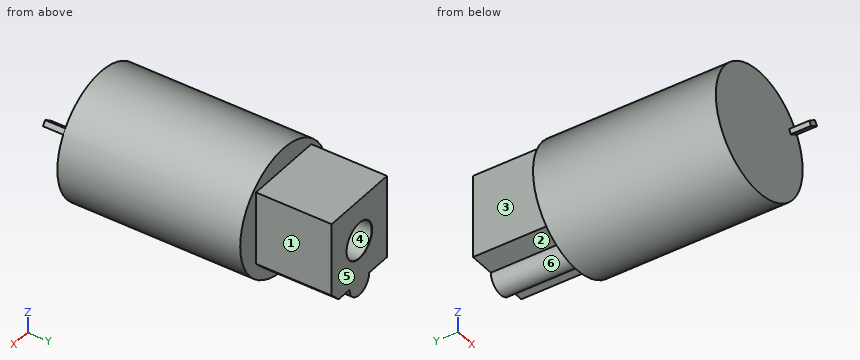
from build123d import *

# Parameters (mm, degrees)
ESBO_O1_R                              = 6.2
RESSALTO_EXTRUS_O1_DEPTH               = 18.1
RESSALTO_EXTRUS_O2_DEPTH               = 2
RESSALTO_EXTRUS_O3_DEPTH               = 7.5
CHANFRO1_SIZE                          = 1
FURO_DE_DI_METRO_3_6_3_6_1_D           = 3.6
FURO_DE_DI_METRO_3_6_3_6_1_DEPTH       = 10
FURO_DE_DI_METRO_3_6_3_6_1_CSINK_D     = 3.65
FURO_DE_DI_METRO_3_6_3_6_1_CSINK_ANGLE = 90
FURO_DE_DI_METRO_3_6_3_6_1_TIP         = 1.081549114


with BuildPart() as part:
    # Esboço1 → Ressalto-extrusão1 (new body)
    with BuildSketch(Plane(origin=(0, 0, 0), x_dir=(1, 0, 0), z_dir=(0, 1, 0))):
        Circle(ESBO_O1_R)
    extrude(amount=RESSALTO_EXTRUS_O1_DEPTH)

    # Esboço2 → Ressalto-extrusão2 (add)
    with BuildSketch(Plane(origin=(0, 0, 0), x_dir=(1, 0, 0), z_dir=(0, 1, 0))):
        with BuildLine():
            Line((4.5033321, -2.6), (5.369357503, -3.1))
            ThreePointArc((5.369357503, -3.1), (5.229026964, -3.331257572), (5.078742675, -3.556173905))
            Line((5.078742675, -3.556173905), (4.25959063, -2.982597469))
            ThreePointArc((4.25959063, -2.982597469), (4.385635518, -2.793957963), (4.5033321, -2.6))
        make_face()
    extrude(amount=-RESSALTO_EXTRUS_O2_DEPTH)

    # Esboço3 → Ressalto-extrusão3 (add)
    with BuildSketch(Plane(origin=(0, 18.1, 0), x_dir=(1, 0, 0), z_dir=(0, 1, 0))):
        with BuildLine():
            Line((1.4, 4.15), (3.95, 4.15))
            Line((3.95, 4.15), (3.95, -4.15))
            Line((3.95, -4.15), (-3.95, -4.15))
            Line((-3.95, -4.15), (-3.95, 4.15))
            Line((-3.95, 4.15), (-1.4, 4.15))
            ThreePointArc((-1.4, 4.15), (0, 5.55), (1.4, 4.15))
        make_face()
    extrude(amount=RESSALTO_EXTRUS_O3_DEPTH)

    # Chanfro1
    chanfro1_edges = [part.edges().sort_by_distance(p)[0] for p in [
        (3.95, 21.85, -4.15),
    ]]
    chamfer(chanfro1_edges, length=CHANFRO1_SIZE)

    # Furo de diâmetro Ø3.6 (3.6)1
    with Locations(Plane(origin=(0, 25.6, 0), x_dir=(1, 0, 0), z_dir=(0, 1, 0))):
        with Locations((0, 0)):
            CounterSinkHole(FURO_DE_DI_METRO_3_6_3_6_1_D / 2, FURO_DE_DI_METRO_3_6_3_6_1_CSINK_D / 2, depth=FURO_DE_DI_METRO_3_6_3_6_1_DEPTH, counter_sink_angle=FURO_DE_DI_METRO_3_6_3_6_1_CSINK_ANGLE)
            with Locations((0, 0, -(FURO_DE_DI_METRO_3_6_3_6_1_DEPTH + FURO_DE_DI_METRO_3_6_3_6_1_TIP / 2))):  # 118° drill point
                Cone(0, FURO_DE_DI_METRO_3_6_3_6_1_D / 2, FURO_DE_DI_METRO_3_6_3_6_1_TIP, mode=Mode.SUBTRACT)


solid = part.part
Part model, mm, in its own coordinate system. Face numbers are marked on the shaded views. A direction names the side the tool comes from. Coordinates: 2 decimals unless noted, no trailing zeros. Write each loop counter-clockwise with the first axis right and the second up, starting at its lowest first coordinate (ties: lowest second). Pieces come first, ordered by that corner, then holes. Notation, with made-up numbers: (71.5, 76.5) - (128.5, 76.5) arc R20 cw to (128.5, 94.5) - close; hole circle Ø9 at (-30.75, -1). An arc over 180 degrees is marked (long way). Put each result on its own line as item: value.
1. Two-plate mould, pull along X, no slides. Class the marked faces 4, 5 and 6: +X half, -X half, draft (parallel to the pull), parting line (faces both ways), or undercut.
Final values:
face 4: undercut
face 5: draft
face 6: parting line
2. Band-saw the part on B-B (y = 13.5). Write the cut outline in (x, z).
Final values:
outline: circle Ø12.4 at (0, 0)
3. Flat gauge pins, fed straight in: pin 1 Ø0.8 at (x, y) = (2, 22.5) entering from -Z; pin 2 Ø4 at (x, y) = (-1.5, 22) entering from +Z; pin 3 Ø1 at (x, y) = (3.5, 9.5) entering from -Z; pin 4 Ø2 at (x, y) = (5, 22.5) entering from -Z. Where does each tip first touch, or does it go through?
Final values:
pin 1: stops at z = -4.15
pin 2: stops at z = 4.15
pin 3: stops at z = -5.43
pin 4: passes through
4. 3-axis set-ups, long thin cutter, end or side, ignore diameter. For the marked faces 1, 2 and 3: which of +Z, -Z, +X, -X, +Y, -Y reach the whole face in a straight line?
Final values:
face 1: +Z, -Z, +X, +Y
face 2: -Z, -X, +Y
face 3: +Z, -Z, -X, +Y
5. Probe line 1 along Z through (x, y) = (0, 23.5); line 2 along Z through (x, y) = (0, 18); line 3 along Y through (x, z) = (3.25, 3). List the from-to ranges inside material, lowest first. Write a range as [from, to].
Final values:
line 1: z = [-5.55, -1.8], [1.8, 4.15]
line 2: z = [-6.2, -1.8], [1.8, 6.2]
line 3: y = [0, 25.6]
6. Band-saw the part on A-A (y = 23.75). Write the cut outline in (x, z).
Final values:
outline: (-3.95, -4.15) - (-1.4, -4.15) arc R1.4 ccw to (1.4, -4.15) - (2.95, -4.15) - (3.95, -3.15) - (3.95, 4.15) - (-3.95, 4.15) - close; hole circle Ø3.6 at (0, 0)
